Answer from the drawing. Dimensions are ordinates in mm from the lowest x, y and z of the part. A direction names the side the tool comes from. Give positions to 0.01 mm unless a question says otherwise; leave off trailing zeros. Order: outer loops, then holes, each group sorted by start corner. A loop starts at its lowest first (then second) coordinate and runs counter-clockwise, first axis right, second up. Notation, with made-up numbers: (16.25, 3) - (40.25, 3) arc R18 ccw to (40.25, 12) - close; hole circle Ø5 at (9, 47). An arc over 180 degrees is marked (long way). Answer in a Markdown table with one row per item.
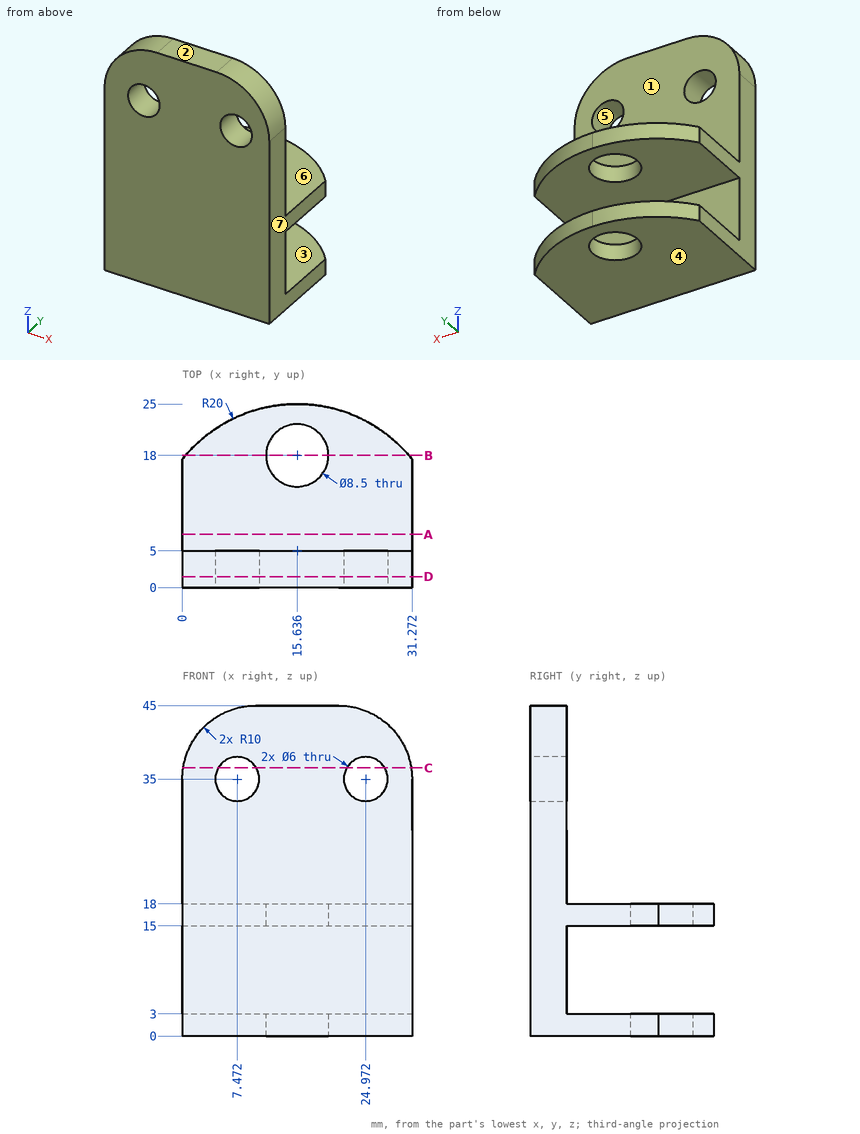
Item 1: Each of these flat-tipped pins is pushed along its axis until it touches: P1, Ø12, axis at y = 11, z = 21, coming from the -X side; P2, Ø6, axis at x = 11, y = 16, coming from the +Z side; P3, Ø7, axis at x = 7.47, z = 35, coming from the +Y side. Where does it stop, or does it pass through?
Answer block:
| item | result |
|---|---|
| P1 | x = 0 |
| P2 | z = 18 |
| P3 | y = 5 |
Item 2: Find section A-A on y = 7.25. Write down the section's boundary in (x, z).
Answer block:
| item | result |
|---|---|
| outline | (0, 0) - (31.27, 0) - (31.27, 3) - (0, 3) - close; (0, 15) - (31.27, 15) - (31.27, 18) - (0, 18) - close |
Item 3: Find section D-D on y = 1.5. Write down the section's boundary in (x, z).
Answer block:
| item | result |
|---|---|
| outline | (0, 0) - (31.27, 0) - (31.27, 35) arc R10 ccw to (21.27, 45) - (10, 45) arc R10 ccw to (0, 35) - close; hole circle Ø6 at (7.47, 35); hole circle Ø6 at (24.97, 35) |
Item 4: Which of the six approach directions +Z, -Z, +X, -X, +Y, -Y give full straight-line access (tool end or side, diameter ignored) to the marked faces 1, 2 and 3?
Answer block:
| item | result |
|---|---|
| face 1 | +Z, +X, -X, +Y |
| face 2 | +Z, +X, -X, +Y, -Y |
| face 3 | +X, -X, +Y |
Item 5: Determine the mould class of the marked faces 4, 5, 6 and 7 for opening direction Z: pulls with the +Z half, pulls with the -Z half, needs draft (parallel to the pull), parting line crosses it, or undercut.
Answer block:
| item | result |
|---|---|
| face 4 | pulls with the -Z half |
| face 5 | undercut |
| face 6 | pulls with the +Z half |
| face 7 | needs draft |
Item 6: Find section B-B on y = 18. Write down the section's boundary in (x, z) (1 decimal).
Answer block:
| item | result |
|---|---|
| outline | (0.4, 0) - (11.4, 0) - (11.4, 3) - (0.4, 3) - close; (0.4, 15) - (11.4, 15) - (11.4, 18) - (0.4, 18) - close; (19.9, 0) - (30.8, 0) - (30.8, 3) - (19.9, 3) - close; (19.9, 15) - (30.8, 15) - (30.8, 18) - (19.9, 18) - close |
Item 7: Find section C-C on z = 36.5. Write down the section's boundary in (x, y).
Answer block:
| item | result |
|---|---|
| outline | (0.11, 0) - (4.87, 0) - (4.87, 5) - (0.11, 5) - close; (10.07, 0) - (22.37, 0) - (22.37, 5) - (10.07, 5) - close; (27.57, 0) - (31.16, 0) - (31.16, 5) - (27.57, 5) - close |
Item 8: Consider line 1 (X direction, y = 1.25, z = 35); line 2 (Z direction, x = 11, y = 12); line 3 (X direction, y = 4, z = 34.5). Determine where each line is inside the solid, lowest interval first.
Answer block:
| item | result |
|---|---|
| line 1 | 0 to 4.47, 10.47 to 21.97, 27.97 to 31.27 |
| line 2 | 0 to 3, 15 to 18 |
| line 3 | 0 to 4.51, 10.43 to 22.01, 27.93 to 31.27 |
